Design review of the part built by this model. Coordinates are the model's own, in mm. Face numbers are marked on the shaded views. A direction names the side the tool comes from. Round coordinates to 2 decimals unless told otherwise and drop trailing zeros. Loops run counter-clockwise (first coordinate to the right, second up) from the corner with the lowest first, then second, coordinate; pieces in that order, holes last. Notation, with made-up numbers: (31, 89.5) - (88, 89.5) arc R34 ccw to (88, 119.5) - close; hole circle Ø8 at (8.5, -31.5). An arc over 180 degrees is marked (long way). Use one line per item in the form item = value. Start each with the question number.
(1) We need section C-C, the plane y = -2. Write out the cut boundary in (x, z).
(2) For pin 1 (2 mm diameter, centred on y = 2.5, z = 0, fed in from +X); pin 2 (5 mm diameter, centred on x = -3.5, y = -3.5, fed in from +Z); pin 3 (1 mm diameter, centred on x = -2, z = 12, fed in from +Y); pin 4 (6 mm diameter, centred on y = 0.5, z = 4.5, fed in from +X), all flat-tipped, find the tip position at first contact; note any pin that passes through.
(3) We need section D-D, the plane z = 3.25. Write out the cut boundary in (x, y).
(4) Wall thickness on probe 1 along Z at (x, y) = (1, 1.75); probe 2 along Z at (x, y) = (-3.5, 4.5); probe 3 along Y at (x, z) = (-1.5, 15): over which ranges is each line inside the solid? List them lowest first. Write a range as [from, to].
(5) Machinability: for the marked faces 1 and 2, which of the approach directions +Z, -Z, +X, -X, +Y, -Y give a long, thin tool a straight path to every point of the face, cutting with its end or side? Answer none if there is none.
(6) We need section A-A, the plane y = 0. Write out the cut boundary in (x, z), then the cut area to 3 significant figures.
from build123d import *

# Parameters (mm, degrees)
F0_W = 1.75
F0_H = 1.25


with BuildPart() as f1:
    # F0 (on Front) → F1 (revolve)
    with BuildSketch(Plane.XZ):
        with Locations((-0.875, 13.125)):
            Rectangle(F0_W, F0_H)
        Polygon((-2.25, 16.25), (-2.25, 13.75), (-1.75, 13.75), (0, 13.75), (0, 16.25), align=None)
        Polygon((-2.25, 12.5), (-2.25, 3.75), (0, 3.75), (0, 12.5), (-1.75, 12.5), align=None)
        Polygon((-2.25, 3.75), (-6, 3.75), (-6, -3.75), (0, -3.75), (0, 3.75), align=None)
    revolve(axis=Axis((0, 0, 6.25), (0, 0, 1)))


solid = f1.part
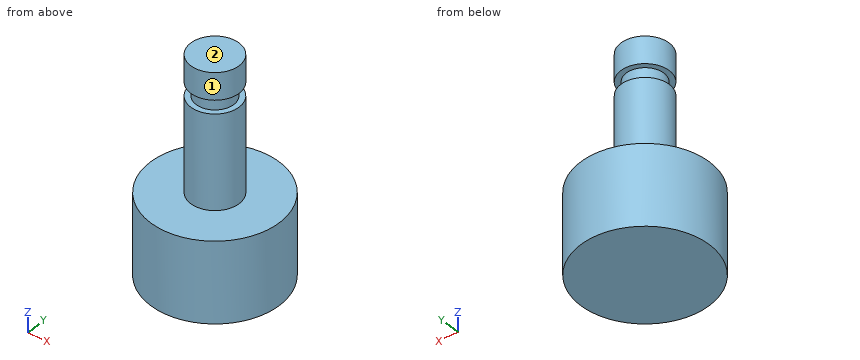
Data:
q1.outline = (-5.66, -3.75) - (5.66, -3.75) - (5.66, 3.75) - (1.03, 3.75) - (1.03, 12.5) - (-1.03, 12.5) - (-1.03, 3.75) - (-5.66, 3.75) - close; (-1.03, 13.75) - (1.03, 13.75) - (1.03, 16.25) - (-1.03, 16.25) - close
q2.pin_1 = 5.81
q2.pin_2 = 3.75
q2.pin_3 = 1.68
q2.pin_4 = 6
q3.outline = circle Ø12 at (0, 0)
q4.probe_1 = [-3.75, 12.5], [13.75, 16.25]
q4.probe_2 = [-3.75, 3.75]
q4.probe_3 = [-1.68, 1.68]
q5.face_1 = +Z
q5.face_2 = +Z, +X, -X, +Y, -Y
q6.outline = (-6, -3.75) - (6, -3.75) - (6, 3.75) - (2.25, 3.75) - (2.25, 12.5) - (1.75, 12.5) - (1.75, 13.75) - (2.25, 13.75) - (2.25, 16.25) - (-2.25, 16.25) - (-2.25, 13.75) - (-1.75, 13.75) - (-1.75, 12.5) - (-2.25, 12.5) - (-2.25, 3.75) - (-6, 3.75) - close
q6.area = 145 mm^2
